Read the model definition and answer for the solid it produces. Units are mm, in the model's axes. Face numbers are marked on the shaded views. A direction names the side the tool comes from. Give positions to 0.01 mm unless a question says otherwise; leave off trailing zeros. Loops run counter-clockwise (first coordinate to the right, second up) from the corner with the lowest first, then second, coordinate; pieces in that order, holes last. Notation, with made-up numbers: M 20.25,66 L 56.25,66 A35 ccw 56.25,100 Z; hole C -18,58 d3. An arc over 180 degrees is marked long. Return JSON: item names as keys, results as strings. Group by question number.
```python
from build123d import *

# Parameters (mm, degrees)
SKETCH_1_R             = 5.5
EXTRUDE_1_DEPTH        = 72
CHAMFER_1_SIZE         = 0.5
SKETCH_2_R             = 3.3
EXTRUDE_2_DEPTH        = 8
HOLE_WIZARD_M5_1_D     = 4.2
HOLE_WIZARD_M5_1_DEPTH = 12.4
HOLE_WIZARD_M5_1_TIP   = 1.2618073
CHAMFER_3_SIZE         = 0.5
SKETCH_6_W             = 10
SKETCH_6_H             = 3
CUT_EXTRUDE_1_DEPTH    = 13


# Read off the part's stored shape, not the designer's step: M6 机械螺纹 螺柱1
with BuildPart() as part:
    # 草图1 → 拉伸1 (new body)
    with BuildSketch(Plane.XY):
        Circle(SKETCH_1_R)
    extrude(amount=EXTRUDE_1_DEPTH)

    # 倒角1
    chamfer_1_edges = [part.edges().sort_by_distance(p)[0] for p in [
        (-5.5, 0, 0),
        (-5.5, 0, 72),
    ]]
    chamfer(chamfer_1_edges, length=CHAMFER_1_SIZE)

    # 草图2 → 拉伸2 (add)
    with BuildSketch(Plane.XY.offset(72)):
        Circle(SKETCH_2_R)
    extrude(amount=EXTRUDE_2_DEPTH)

    # M5 螺纹孔1
    with Locations(Plane(origin=(0, 0, 0), x_dir=(-1, 0, 0), z_dir=(0, 0, -1))):
        with Locations((0, 0)):
            Hole(HOLE_WIZARD_M5_1_D / 2, depth=HOLE_WIZARD_M5_1_DEPTH)
            with Locations((0, 0, -(HOLE_WIZARD_M5_1_DEPTH + HOLE_WIZARD_M5_1_TIP / 2))):  # 118° drill point
                Cone(0, HOLE_WIZARD_M5_1_D / 2, HOLE_WIZARD_M5_1_TIP, mode=Mode.SUBTRACT)

    # 倒角3
    chamfer_3_edges = [part.edges().sort_by_distance(p)[0] for p in [
        (-2.1, 0, 0),
    ]]
    chamfer(chamfer_3_edges, length=CHAMFER_3_SIZE)

    # 草图6 → 切除-拉伸1 (cut)
    with BuildSketch(Plane(origin=(0, 0, 0), x_dir=(-1, 0, 0), z_dir=(0, 0, -1))):
        with Locations((0, 6.5)):
            Rectangle(SKETCH_6_W, SKETCH_6_H)
        with Locations((0, -6.5)):
            Rectangle(SKETCH_6_W, SKETCH_6_H)
    extrude(amount=-CUT_EXTRUDE_1_DEPTH, mode=Mode.SUBTRACT)

    # M6 机械螺纹 螺柱1 outline → M6 机械螺纹 螺柱1 (revolve, cut)
    with BuildSketch(Plane.XZ):
        Polygon((3.3, 80), (2.4585, 80), (3, 79.4585), (3, 72), (3.3, 72), align=None)
    revolve(axis=Axis((0, 0, 0), (0, 0, 1)), mode=Mode.SUBTRACT)


solid = part.part
```
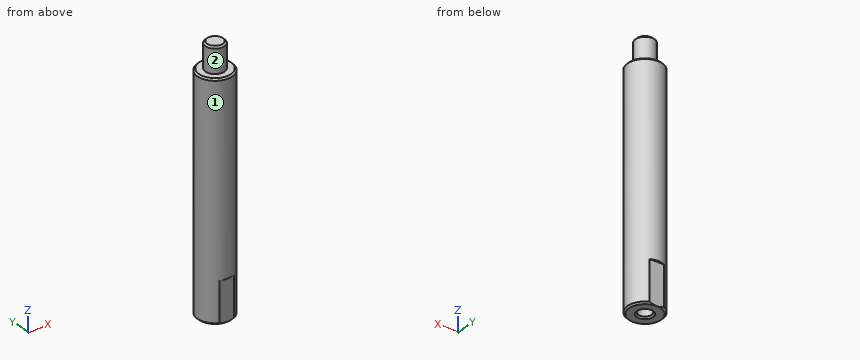
1. Find section B-B (z = 74.5). Write down the section's boundary in (x, y), and give its area (3 significant figures).
2. Find section A-A (z = 33.5). Write down the section's boundary in (x, y), and give its area (3 significant figures).
3. For the marked faces 1 and 2, determine the directions among +Z, -Z, +X, -X, +Y, -Y from which every point of the face is accessible in a straight line to the end or side of a thin tool.
4. Flat-ended cylindrical pins translate along their axes: P1, Ø1, axis at x = -2, z = 65, coming from the -Y side; P2, Ø1.4, axis at x = 0, z = 6.5, coming from the +Y side; P3, Ø1, axis at x = 3.5, z = 53, coming from the -Y side. Find the tip coordinate at first contact, or state that the pin passes through.
5. Straight lines are drawn through the part: line 1 along Y through (x, z) = (0, 7.25); line 2 along X through (y, z) = (0, 8); line 3 along Z through (x, y) = (-2, -3.5). For each, find the intervals that lie inside material, in ascending order.
Result:
{
 "1": {"outline": "C 0,0 d6", "area": "28.3 mm2"},
 "2": {"outline": "C 0,0 d11", "area": "95.0 mm2"},
 "3": {"face 1": "+Z, -Z", "face 2": "+Z"},
 "4": {"P1": "stops at y = -5.29", "P2": "stops at y = 5", "P3": "stops at y = -4.61"},
 "5": {"line 1": "y = -5 to -2.1, 2.1 to 5", "line 2": "x = -5.5 to -2.1, 2.1 to 5.5", "line 3": "z = 0 to 72"}
}
